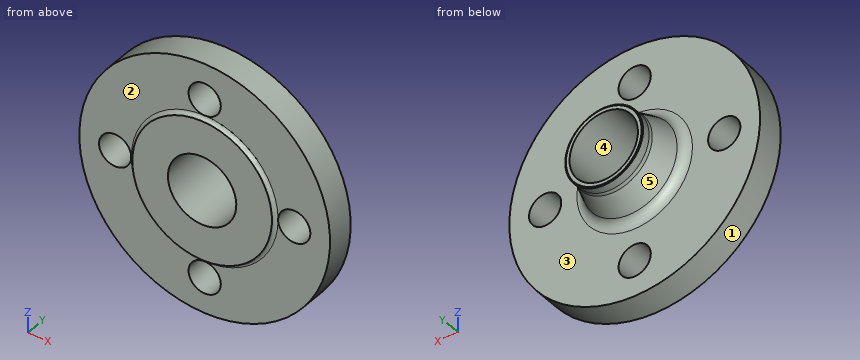
Autodesk Inventor part; units mm, degrees
ref_plane "YZ Plane" through (0, 0, 0) normal (1, 0, 0) x (0, 1, 0)
ref_plane "XZ Plane" through (0, 0, 0) normal (0, 1, 0) x (-1, 0, 0)
ref_plane "XY Plane" through (0, 0, 0) normal (0, 0, 1) x (1, 0, 0)
sketch "Sketch1" plane through (0, 0, 0) normal (1, 0, 0) x (0, 1, 0)
  line L0 (0, 0) -> (150, 0)
  line L1 (0, 0) -> (0, 39)
  line L2 (0, 39) -> (2, 39)
  line L3 (2, 39) -> (2, 70)
  line L4 (2, 70) -> (18, 70)
  line L5 (18, 70) -> (18, 28)
  line L6 (18, 28) -> (36, 21.75)
  line L7 (36, 21.75) -> (42, 21.75)
  line L8 (42, 21.75) -> (42, 0)
  dimension "d0" = 150
  dimension "d1" = 78
  dimension "d2" = 140
  dimension "d3" = 56
  dimension "d4" = 43.5
  dimension "d5" = 2
  dimension "d6" = 18
  dimension "d7" = 6
  dimension "d8" = 42
revolve "Revolution1" add sketch "Sketch1" angle 360 about axis through (0, 0, 0) along (0, 1, 0)
fillet "Fillet1" radius 2 1 edges at (0, 2, -39)
fillet "Fillet2" radius 6 2 edges at (0, 18, -28) (0, 36, -21.75)
chamfer "Chamfer1" distance 0.6 angle 30 1 edges at (0, 42, -21.75) measured on face at (-7.8802, 42, -7.0393)
sketch "Sketch2" plane through (0, 18, 0) normal (0, 1, 0) x (1, 0, 0)
  point P0 (0, 0)
  point P1 (-50, 0)
  point P2 (0, 50)
  point P3 (50, 0)
  point P4 (0, -50)
hole "Hole1" at (-50, 18, 0) at (0, 18, -50) at (50, 18, 0) at (0, 18, 50) direction (0, -1, 0) diameter 18 end through all
sketch "Sketch4" plane through (0, 42, 0) normal (0, 1, 0) x (1, 0, 0)
  point P0 (0, 0)
  point P1 (0, 0)
hole "Hole2" at (0, 42, 0) direction (0, -1, 0) diameter 38.2 end through all
properties part number "karima" material "Steel, Alloy"
For this review, take the finished solid that the model builds, in its own axes (mm). Face numbers are marked on the shaded views. A direction names the side the tool comes from. Coordinates: 2 decimals unless noted, no trailing zeros. Order: outer loops, then holes, each group sorted by start corner. A loop starts at its lowest first (then second) coordinate and runs counter-clockwise, first axis right, second up. Notation, with made-up numbers: (78, 31) - (88, 31) arc R28 cw to (88, 56) - close; hole circle Ø7 at (22.5, -24). An arc over 180 degrees is marked (long way). Answer as CSV lines item,"result". Start each with the question number.
1) Insertion check: P1, Ø3, axis at x = 43.5, y = 8.5, coming from the +Z side; P2, Ø6, axis at x = -49.5, y = 18, coming from the +Z side; P3, Ø23.5, axis at x = -50, z = 0, coming from the +Y side. Each pin has a flat end and moves straight along its axis. Give the tip position at first contact, or say it passes through.
2) Add section C-C (y = 9). State the section outline as (x, z) points, then the cut area to 3 significant figures.
3) Draft analysis for pull direction Z (two halves, no side actions). For the marked faces 3, 4 and 5, state which applies: +Z half, -Z half, draft (parallel to the pull), parting line (faces both ways), or undercut.
4) To check wall thickness, follow line 1 along X through (y, z) = (8, 0); line 2 along Y through (x, z) = (32, 29.5); line 3 along X through (y, z) = (18.5, 2) (3 decimals). State the ranges of each line that lie inside material, in increasing order. Write a range as [from, to].
5) Add section B-B (x = 50). State the section outline as (y, z) points.
6) Add section D-D (z = 0). Count the separate pieces of the cut face and the enclosed holes in it, then the cut area to 3 significant figures.
7) Add section A-A (z = 50). State the section outline as (x, y) points.
8) Machinability: for the marked faces 1 and 2, which of the approach directions +Z, -Z, +X, -X, +Y, -Y give a long, thin tool a straight path to every point of the face, cutting with its end or side? Answer none if there is none.
Result:
1,P1,"z = 56"
1,P2,"z = 52.32"
1,P3,"y = 18"
2,outline,"circle Ø140 at (0, 0); hole circle Ø18 at (-50, 0); hole circle Ø38.2 at (0, 0); hole circle Ø18 at (0, -50); hole circle Ø18 at (0, 50); hole circle Ø18 at (50, 0)"
2,area,"13,200 mm^2"
3,face 3,"draft"
3,face 4,"undercut"
3,face 5,"parting line"
4,line 1,"[-70, -59], [-41, -19.1], [19.1, 41], [59, 70]"
4,line 2,"[2, 18]"
4,line 3,"[-29.803, -18.995], [18.995, 29.803]"
5,outline,"(2, -48.99) - (18, -48.99) - (18, -9) - (2, -9) - close; (2, 9) - (18, 9) - (18, 48.99) - (2, 48.99) - close"
6,separate pieces,"4"
6,enclosed holes,"0"
6,area,"1,380 mm^2"
7,outline,"(-48.99, 2) - (-9, 2) - (-9, 18) - (-48.99, 18) - close; (9, 2) - (48.99, 2) - (48.99, 18) - (9, 18) - close"
8,face 1,"+Y, -Y"
8,face 2,"-Y"
